Work out the finished part from the listing and answer in its coordinate system (mm). Face numbers are marked on the shaded views. A direction names the side the tool comes from. Round coordinates to 2 decimals unless told otherwise and drop trailing zeros. Loops run counter-clockwise (first coordinate to the right, second up) from the corner with the lowest first, then second, coordinate; pieces in that order, holes last. Notation, with made-up numbers: (22, 75.5) -> (43, 75.5) arc R35 cw to (43, 111.5) -> close; hole circle Ø7 at (71.5, 7.25). An arc over 180 degrees is marked (long way). Write item = value, one per line. Start each with the question number.
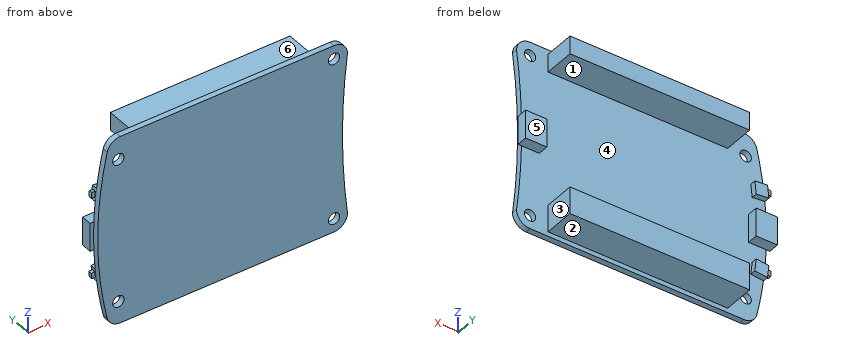
```python
from build123d import *

# Parameters (mm, degrees)
SKETCH1_R           = 1.6
BOSS_EXTRUDE1_DEPTH = 1.6
SKETCH2_W           = 6
SKETCH2_H           = 8
BOSS_EXTRUDE2_DEPTH = 3
BOSS_EXTRUDE3_DEPTH = 1.6
SKETCH4_W           = 1.6
SKETCH4_H           = 1
BOSS_EXTRUDE4_DEPTH = 1
SKETCH5_W           = 1.6
SKETCH5_H           = 1
BOSS_EXTRUDE5_DEPTH = 1
SKETCH6_W           = 50.8
SKETCH6_H           = 5.08
SKETCH6_H_2         = 7.62
BOSS_EXTRUDE6_DEPTH = 8.7


with BuildPart() as part:
    # Sketch1 → Boss-Extrude1 (new body)
    with BuildSketch(Plane(origin=(0, 0, 0), x_dir=(1, 0, 0), z_dir=(0, 1, 0))):
        with BuildLine():
            Line((30.48, 26.67), (-29.941284627, 26.67))
            ThreePointArc((-29.941284627, 26.67), (-32.31004746, 25.841357037), (-33.645726791, 23.716822443))
            ThreePointArc((-33.645726791, 23.716822443), (-36.322, 0), (-33.645726791, -23.716822443))
            ThreePointArc((-33.645726791, -23.716822443), (-32.31004746, -25.841357037), (-29.941284627, -26.67))
            Line((-29.941284627, -26.67), (30.48, -26.67))
            ThreePointArc((30.48, -26.67), (33.174076836, -25.554076836), (34.29, -22.86))
            ThreePointArc((34.29, -22.86), (32.868, 0), (34.29, 22.86))
            ThreePointArc((34.29, 22.86), (33.174076836, 25.554076836), (30.48, 26.67))
        make_face()
        with Locations((30.48, 22.86)):
            Circle(SKETCH1_R, mode=Mode.SUBTRACT)
        with Locations((-30.48, 20.32)):
            Circle(SKETCH1_R, mode=Mode.SUBTRACT)
        with Locations((30.48, -22.86)):
            Circle(SKETCH1_R, mode=Mode.SUBTRACT)
        with Locations((-30.48, -20.32)):
            Circle(SKETCH1_R, mode=Mode.SUBTRACT)
    extrude(amount=BOSS_EXTRUDE1_DEPTH)

    # Sketch2 → Boss-Extrude2 (add)
    with BuildSketch(Plane(origin=(0, 1.6, 0), x_dir=(1, 0, 0), z_dir=(0, 1, 0))):
        with Locations((-34.322, 0)):
            Rectangle(SKETCH2_W, SKETCH2_H)
        with Locations((30.868, 0)):
            Rectangle(SKETCH2_W, SKETCH2_H)
    extrude(amount=BOSS_EXTRUDE2_DEPTH)

    # Sketch3 → Boss-Extrude3 (add)
    with BuildSketch(Plane(origin=(0, 1.6, 0), x_dir=(1, 0, 0), z_dir=(0, 1, 0))):
        Polygon((-35.510618925, 13.239552311), (-31.931514302, 12.85224094), (-32.318825673, 9.273136317), (-35.897930296, 9.660447689), align=None)
        Polygon((-31.931514302, -12.85224094), (-32.318825673, -9.273136317), (-35.897930296, -9.660447689), (-35.510618925, -13.239552311), align=None)
    extrude(amount=BOSS_EXTRUDE3_DEPTH)

    # Sketch4 → Boss-Extrude4 (add)
    with BuildSketch(Plane(origin=(-36.515718124, 0, 3.951533791), x_dir=(0.107586492, 0, 0.994195729), z_dir=(-0.994195729, 0, 0.107586492))):
        with Locations((7.542243437, 2.4)):
            Rectangle(SKETCH4_W, SKETCH4_H)
    extrude(amount=BOSS_EXTRUDE4_DEPTH)

    # Sketch5 → Boss-Extrude5 (add)
    with BuildSketch(Plane(origin=(-36.515718124, 0, -3.951533791), x_dir=(-0.107586492, 0, 0.994195729), z_dir=(-0.994195729, 0, -0.107586492))):
        with Locations((-7.542243437, 2.4)):
            Rectangle(SKETCH5_W, SKETCH5_H)
    extrude(amount=BOSS_EXTRUDE5_DEPTH)

    # Sketch6 → Boss-Extrude6 (add)
    with BuildSketch(Plane(origin=(0, 1.6, 0), x_dir=(1, 0, 0), z_dir=(0, 1, 0))):
        with Locations((0, -22.86)):
            Rectangle(SKETCH6_W, SKETCH6_H)
        with Locations((0, 21.59)):
            Rectangle(SKETCH6_W, SKETCH6_H_2)
    extrude(amount=BOSS_EXTRUDE6_DEPTH)


solid = part.part
```
Item 1: Section B-B (z = -20.32) is taken. Determine the outline of the cut face in (x, y), then the cut area to 3 significant figures.
Item 2: Section D-D (z = 8) is taken. Determine the outline of the cut face in (x, y).
Item 3: The mould has two halves that part along Z. Classify the marked faces 4, 5 and 6: pulls with the +Z half, pulls with the -Z half, needs draft (parallel to the pull), parting line crosses it, or undercut.
Item 4: A tool of negligible diameter and unlimited length cuts with its end or side. For the marked faces 1, 2 and 3, from which of +Z, -Z, +X, -X, +Y, -Y can it reach the whole face along a straight path? Write none if from no direction.
Item 5: Flat-ended cylindrical pins translate along their axes: pin 1 (2 mm diameter, centred on y = 1, z = 15, fed in from -X); pin 2 (3 mm diameter, centred on x = 4, z = 19, fed in from +Y); pin 3 (3 mm diameter, centred on x = -33.5, z = -12, fed in from +Y); pin 4 (0.8 mm diameter, centred on x = 33.5, z = 0, fed in from -Y). Find the tip coordinate at first contact, or state that the pin passes through.
Item 6: Section C-C (x = 11) is taken. Determine the outline of the cut face in (y, z), then the cut area to 3 significant figures.
Item 7: Section A-A (y = 7.75) is taken. Determine the outline of the cut face in (x, z).
Item 8: Find the intervals of material crossed by line 1 along Z through (x, y) = (30.48, 1.3); line 2 along Z through (x, y) = (-21.5, 5.75); line 3 along Y through (x, z) = (19.5, 3.5), in increasing order. Write a range as [from, to].
Worked answers:
q1.outline = (-34.36, 0) -> (-32.08, 0) -> (-32.08, 1.6) -> (-34.36, 1.6) -> close; (-28.88, 0) -> (33.99, 0) -> (33.99, 1.6) -> (25.4, 1.6) -> (25.4, 10.3) -> (-25.4, 10.3) -> (-25.4, 1.6) -> (-28.88, 1.6) -> close
q1.area = 546 mm2
q2.outline = (-36.02, 0) -> (33.04, 0) -> (33.04, 1.6) -> (-36.02, 1.6) -> close
q3.face_4 = undercut
q3.face_5 = needs draft
q3.face_6 = pulls with the +Z half
q4.face_1 = +X, -X, +Y
q4.face_2 = -Z, +X, -X, +Y
q4.face_3 = +Z, -Z, +X, +Y
q5.pin_1 = -35.4
q5.pin_2 = 10.3
q5.pin_3 = 3.2
q5.pin_4 = 1.6
q6.outline = (0, -26.67) -> (1.6, -26.67) -> (1.6, -25.4) -> (10.3, -25.4) -> (10.3, -17.78) -> (1.6, -17.78) -> (1.6, 20.32) -> (10.3, 20.32) -> (10.3, 25.4) -> (1.6, 25.4) -> (1.6, 26.67) -> (0, 26.67) -> close
q6.area = 196 mm2
q7.outline = (-25.4, -25.4) -> (25.4, -25.4) -> (25.4, -17.78) -> (-25.4, -17.78) -> close; (-25.4, 20.32) -> (25.4, 20.32) -> (25.4, 25.4) -> (-25.4, 25.4) -> close
q8.line_1 = [-26.67, -24.46], [-21.26, 21.26], [24.46, 26.67]
q8.line_2 = [-25.4, -17.78], [20.32, 25.4]
q8.line_3 = [0, 1.6]
